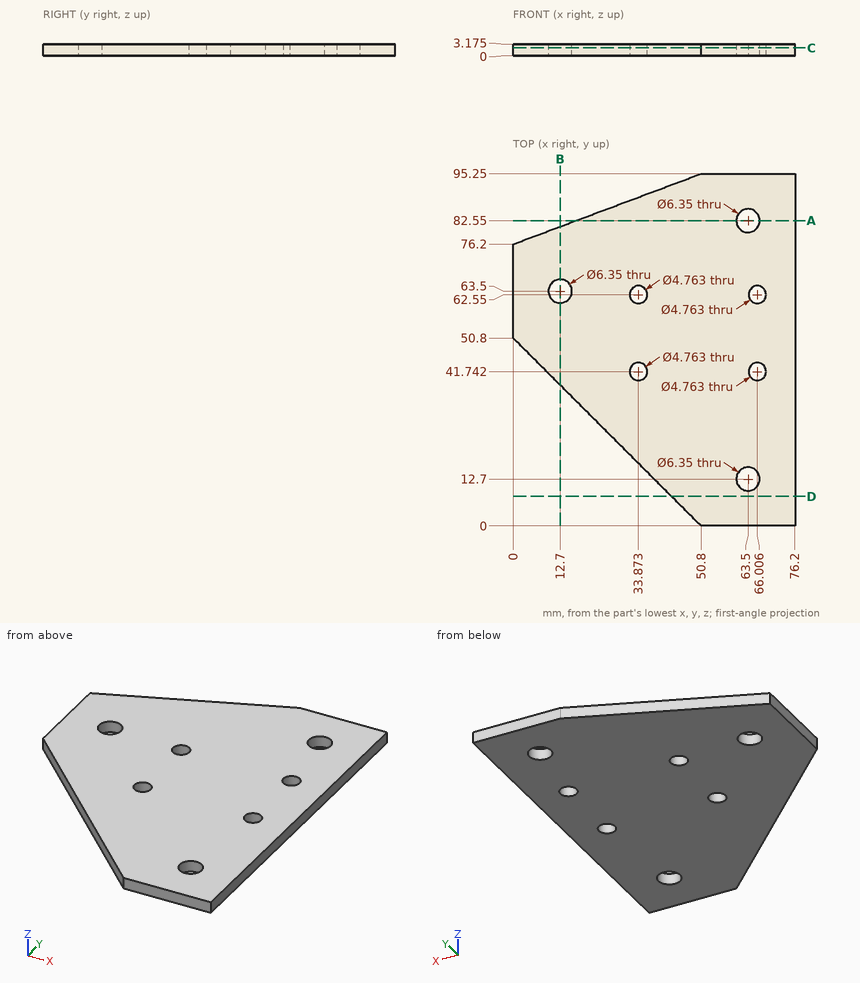
Part print with two shaded views. Sizes in mm from the minimum x, y, z corner. Coordinates: 2 decimals unless noted, no trailing zeros. Loops run counter-clockwise (first coordinate to the right, second up) from the corner with the lowest first, then second, coordinate; pieces in that order, holes last. Notation, with made-up numbers: (60, 55) - (71, 55) arc R12 ccw to (71, 69) - close; hole circle Ø6 at (-25, -37.5). An arc over 180 degrees is marked (long way). Write each question's results on one line, items separated by ' | '. Start each with the question number.
Q1. Slice it at A-A on y = 82.55. Give the cut face in (x, z) (1 decimal).
Q2. Drop flat-ended pins along their axis: pin 1 Ø1 at (y, z) = (39.5, 2.5) entering from -X; pin 2 Ø1 at (x, z) = (41, 2) entering from -Y. Give the stop position or say it passes through.
Q3. Slice it at C-C on z = 2.15. Give the number of separate pieces and of enclosed holes in the cut face, and give its area (3 significant figures).
Q4. Probe line 1 along Y through (x, z) = (11.5, 0.25); line 2 along Y through (x, z) = (50, 0.75); line 3 along Y through (x, z) = (28.5, 1.65). List the from-to ranges inside material, lowest first.
Q5. Slice it at D-D on y = 8. Give the cut face in (x, z) (1 decimal), and give its area (3 significant figures).
Q6. Slice it at B-B on x = 12.7. Give the cut face in (y, z) (1 decimal).
Answer:
1) outline: (16.9, 0) - (60.3, 0) - (60.3, 3.2) - (16.9, 3.2) - close; (66.7, 0) - (76.2, 0) - (76.2, 3.2) - (66.7, 3.2) - close
2) pin 1: stops at x = 10.8 | pin 2: stops at y = 9.3
3) separate pieces: 1 | enclosed holes: 7 | area: 5,320 mm2
4) line 1: y = 39.3 to 60.56, 66.44 to 80.51 | line 2: y = 0.8 to 94.95 | line 3: y = 22.3 to 86.89
5) outline: (42.8, 0) - (76.2, 0) - (76.2, 3.2) - (42.8, 3.2) - close | area: 106 mm2
6) outline: (38.1, 0) - (60.3, 0) - (60.3, 3.2) - (38.1, 3.2) - close; (66.7, 0) - (81, 0) - (81, 3.2) - (66.7, 3.2) - close
